```python
from build123d import *

# Parameters (mm, degrees)
F1_DEPTH = 19.05


with BuildPart() as f1:
    # F0 (on Front) → F1 (new body)
    with BuildSketch(Plane.XZ):
        with BuildLine():
            add(Edge.make_bspline(
                [(-203.2, 0), (-175.011158, 21.012219), (-135.466667, 8.466667), (-101.6, 12.7)],
                knots=[0, 0, 0, 0, 102.390673, 102.390673, 102.390673, 102.390673], degree=3))
            add(Edge.make_bspline(
                [(-203.2, 0), (-193.597674, -22.507101), (-128.455162, -36.779895), (-82.55, -38.1)],
                knots=[0, 0, 0, 0, 126.522854, 126.522854, 126.522854, 126.522854], degree=3))
            add(Edge.make_bspline(
                [(190.5, -50.8), (99.483333, -46.566667), (-90.760343, -50.8), (-82.55, -38.1)],
                knots=[0, 0, 0, 0, 273.345189, 273.345189, 273.345189, 273.345189], degree=3))
            add(Edge.make_bspline(
                [(203.2, -38.1), (203.11287, -45.563158), (199.453175, -50.686721), (190.5, -50.8)],
                knots=[0, 0, 0, 0, 17.960512, 17.960512, 17.960512, 17.960512], degree=3))
            Line((203.2, -38.1), (203.2, 38.1))
            add(Edge.make_bspline(
                [(203.2, 38.1), (203.478828, 42.635404), (204.576746, 49.588814), (196.85, 50.8)],
                knots=[0, 0, 0, 0, 14.199032, 14.199032, 14.199032, 14.199032], degree=3))
            add(Edge.make_bspline(
                [(196.85, 50.8), (153.912932, 50.8), (160.194486, 25.984986), (127, 0)],
                knots=[0, 0, 0, 0, 86.369338, 86.369338, 86.369338, 86.369338], degree=3))
            Line((127, 0), (63.5, 6.35))
            add(Edge.make_bspline(
                [(0, 19.05), (32.403201, 21.242376), (42.333333, 10.583333), (63.5, 6.35)],
                knots=[0, 0, 0, 0, 64.757548, 64.757548, 64.757548, 64.757548], degree=3))
            Line((0, 19.05), (0, 12.7))
            add(Edge.make_bspline(
                [(-76.2, 25.4), (-50.794795, 31.152328), (-25.4, 16.933333), (0, 12.7)],
                knots=[0, 0, 0, 0, 77.251084, 77.251084, 77.251084, 77.251084], degree=3))
            Line((-76.2, 25.4), (-101.6, 12.7))
        make_face()
    extrude(amount=F1_DEPTH)


solid = f1.part
```
Can you work these out from the model? Positions are in its coordinate system, mm. A direction names the side the tool comes from. Round coordinates to 2 decimals unless told otherwise and drop trailing zeros. Answer as a JSON object with one key per item and string values. Group by question number.
Q1. Please list where these lines run through material, in increasing order: L1, parallel to X at y = -16.75, z = -39; L2, parallel to Z at x = 166.5, y = -12.75; L3, parallel to Z at x = -120, y = -9.5.
Q2. On a 3-axis mill with a long thin cutter (end or side, diameter ignored), from which of +Z, -Z, +X, -X, +Y, -Y can I reach the whole of each face in a straight line? I mean faces 1 (the flat face through (49, -19.05, -11)), 2 (the flat face through (95.69, -9.39, 3.13)). Say none if no direction works.
Q3. Will these pins go through, and if not, where does the flat tip stop? pin 1 (10 mm diameter, centred on x = -63.5, y = -13.5, fed in from +Z); pin 2 (1.5 mm diameter, centred on x = 151.5, y = -3, fed in from +Z); pin 3 (5 mm diameter, centred on y = -11, z = 15.5, fed in from -X).
Q4. We'd pull the mould along X, two halves only. Please class faces 3 (the flat face through (0, -9, 16)), 4 (the flat face through (49, 0, -11)), 5 (the flat face through (203.2, -9, -1)): +X half, -X half, draft (parallel to the pull), parting line (faces both ways), or undercut.
Findings:
{
 "1": {"L1": "x = -82.8 to 203.17", "L2": "z = -49.92 to 43.02", "L3": "z = -34.67 to 11.75"},
 "2": {"face 1": "+Z, -Z, +X, -X, -Y", "face 2": "+Z, +Y, -Y"},
 "3": {"pin 1": "stops at z = 26.75", "pin 2": "stops at z = 27.33", "pin 3": "stops at x = -101"},
 "4": {"face 3": "undercut", "face 4": "draft", "face 5": "+X half"}
}
